Part model, mm, in its own coordinate system. Face numbers are marked on the shaded views. A direction names the side the tool comes from. Give positions to 0.01 mm unless a question says otherwise; leave off trailing zeros. Order: outer loops, then holes, each group sorted by start corner. A loop starts at its lowest first (then second) coordinate and runs counter-clockwise, first axis right, second up.
1. Mould opens along X. For the marked faces 3, 4, 5 and 6 say: +X half, -X half, draft (parallel to the pull), parting line (faces both ways), or undercut.
2. Slice it at C-C on x = 0. List the corners of the cut face in (y, z), and give its area (3 significant figures).
3. Probe line 1 (Z direction, x = 39, y = 9.25); line 2 (Z direction, x = -37.5, y = 12.5); line 3 (X direction, y = 13.25, z = -40). List the from-to ranges inside material, lowest first.
4. Slice it at B-B on z = 0. List the corners of the cut face in (x, y).
5. Drop flat-ended pins along their axis: pin 1 Ø5 at (y, z) = (11, 12) entering from +X; pin 2 Ø0.8 at (x, y) = (2, 0.5) entering from +Z; pin 3 Ø3 at (y, z) = (10, 5) entering from +X; pin 4 Ø0.8 at (y, z) = (1, 2.5) entering from +X. Give the stop position or say it passes through.
6. Which spindle directions (+Z, -Z, +X, -X, +Y, -Y) get a long thin tool onto all of the face, cutting with end or side? Do the marked faces 1 and 2. Say none if no direction does.
7. Slice it at A-A on y = 10.75. Give the number of separate pieces and of enclosed holes in the cut face, and give its area (3 significant figures).
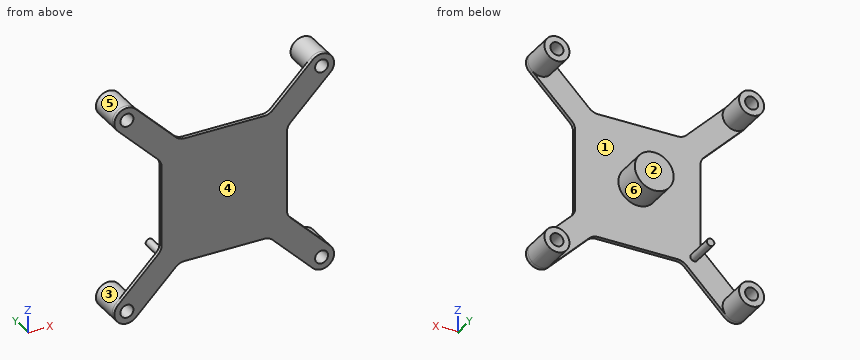
from build123d import *

# Parameters (mm, degrees)
SKETCH1_W           = 50
SKETCH1_H           = 50
SKETCH1_R           = 8
BOSS_EXTRUDE1_DEPTH = 1.5
BOSS_EXTRUDE3_START = -1.5
SKETCH5_R           = 2.6
SKETCH5_R_2         = 8
BOSS_EXTRUDE3_DEPTH = 1.5
FILLET1_R           = 5
SKETCH6_R           = 5
SKETCH6_R_2         = 2.6
BOSS_EXTRUDE4_DEPTH = 12
SKETCH7_R           = 8.25
BOSS_EXTRUDE5_DEPTH = 1.5
SKETCH8_R           = 7.75
BOSS_EXTRUDE6_DEPTH = 12
SKETCH9_R           = 1.5
BOSS_EXTRUDE7_DEPTH = 12


with BuildPart() as part:
    # Sketch1 → Boss-Extrude1 (new body)
    with BuildSketch(Plane(origin=(0, 0, 0), x_dir=(1, 0, 0), z_dir=(0, 1, 0))):
        Rectangle(SKETCH1_W, SKETCH1_H)
        with Locations(Location((0, 0, 0), (0, 0, 270))):
            Circle(SKETCH1_R, mode=Mode.SUBTRACT)
    extrude(amount=BOSS_EXTRUDE1_DEPTH)

    # Sketch5 → Boss-Extrude3 (add)
    with BuildSketch(Plane(origin=(0, 1.5, 0), x_dir=(1, 0, 0), z_dir=(0, 1, 0)).offset(BOSS_EXTRUDE3_START)):
        Polygon((-42.426406871, -35.355339059), (-25, -17.928932188), (-25, 17.928932188), (-42.426406871, 35.355339059), (-45.961940777, 38.890872965), (-38.890872965, 45.961940777), (-35.355339059, 42.426406871), (-17.928932188, 25), (17.928932188, 25), (35.355339059, 42.426406871), (38.890872965, 45.961940777), (45.961940777, 38.890872965), (42.426406871, 35.355339059), (25, 17.928932188), (25, -17.928932188), (42.426406871, -35.355339059), (45.961940777, -38.890872965), (38.890872965, -45.961940777), (35.355339059, -42.426406871), (17.928932188, -25), (-17.928932188, -25), (-35.355339059, -42.426406871), (-38.890872965, -45.961940777), (-45.961940777, -38.890872965), align=None)
        with Locations(Location((-38.890872965, -38.890872965, 0), (0, 0, 270))):
            Circle(SKETCH5_R, mode=Mode.SUBTRACT)
        with Locations(Location((38.890872965, 38.890872965, 0), (0, 0, 270))):
            Circle(SKETCH5_R, mode=Mode.SUBTRACT)
        with Locations(Location((38.890872965, -38.890872965, 0), (0, 0, 90))):
            Circle(SKETCH5_R, mode=Mode.SUBTRACT)
        with Locations(Location((-38.890872965, 38.890872965, 0), (0, 0, 90))):
            Circle(SKETCH5_R, mode=Mode.SUBTRACT)
        with Locations(Location((0, 0, 0), (0, 0, 270))):
            Circle(SKETCH5_R_2, mode=Mode.SUBTRACT)
    extrude(amount=BOSS_EXTRUDE3_DEPTH)

    # Fillet1
    fillet1_edges = [part.edges().sort_by_distance(p)[0] for p in [
        (17.928932188, 0.75, 25),
        (38.890872965, 0.75, 45.961940777),
        (45.961940777, 0.75, 38.890872965),
        (25, 0.75, 17.928932188),
        (25, 0.75, -17.928932188),
        (45.961940777, 0.75, -38.890872965),
        (38.890872965, 0.75, -45.961940777),
        (17.928932188, 0.75, -25),
        (-17.928932188, 0.75, -25),
        (-38.890872965, 0.75, -45.961940777),
        (-45.961940777, 0.75, -38.890872965),
        (-25, 0.75, -17.928932188),
        (-25, 0.75, 17.928932188),
        (-45.961940777, 0.75, 38.890872965),
        (-38.890872965, 0.75, 45.961940777),
        (-17.928932188, 0.75, 25),
    ]]
    fillet(fillet1_edges, radius=FILLET1_R - 0.0001)  # a hair under: the kernel refuses the full size

    # Sketch6 → Boss-Extrude4 (add)
    # profile 1 of 4: a face of its own
    with BuildSketch(Plane(origin=(0, 1.5, 0), x_dir=(1, 0, 0), z_dir=(0, 1, 0))):
        with Locations(Location((-38.890872965, -38.890872965, 0), (0, 0, 270))):
            Circle(SKETCH6_R)
        with Locations(Location((-38.890872965, -38.890872965, 0), (0, 0, 270))):
            Circle(SKETCH6_R_2, mode=Mode.SUBTRACT)
    # profile 2 of 4: a face of its own
    with BuildSketch(Plane(origin=(0, 1.5, 0), x_dir=(1, 0, 0), z_dir=(0, 1, 0))):
        with Locations(Location((-38.890872965, 38.890872965, 0), (0, 0, 270))):
            Circle(SKETCH6_R)
        with Locations(Location((-38.890872965, 38.890872965, 0), (0, 0, 270))):
            Circle(SKETCH6_R_2, mode=Mode.SUBTRACT)
    # profile 3 of 4: a face of its own
    with BuildSketch(Plane(origin=(0, 1.5, 0), x_dir=(1, 0, 0), z_dir=(0, 1, 0))):
        with Locations(Location((38.890872965, 38.890872965, 0), (0, 0, 270))):
            Circle(SKETCH6_R)
        with Locations(Location((38.890872965, 38.890872965, 0), (0, 0, 270))):
            Circle(SKETCH6_R_2, mode=Mode.SUBTRACT)
    # profile 4 of 4: a face of its own
    with BuildSketch(Plane(origin=(0, 1.5, 0), x_dir=(1, 0, 0), z_dir=(0, 1, 0))):
        with Locations(Location((38.890872965, -38.890872965, 0), (0, 0, 270))):
            Circle(SKETCH6_R)
        with Locations(Location((38.890872965, -38.890872965, 0), (0, 0, 270))):
            Circle(SKETCH6_R_2, mode=Mode.SUBTRACT)
    extrude(amount=BOSS_EXTRUDE4_DEPTH)

    # Sketch7 → Boss-Extrude5 (add)
    with BuildSketch(Plane(origin=(0, 1.5, 0), x_dir=(1, 0, 0), z_dir=(0, 1, 0))):
        Circle(SKETCH7_R)
    extrude(amount=-BOSS_EXTRUDE5_DEPTH)

    # Sketch8 → Boss-Extrude6 (add)
    with BuildSketch(Plane(origin=(0, 1.5, 0), x_dir=(1, 0, 0), z_dir=(0, 1, 0))):
        with Locations(Location((0, 0, 0), (0, 0, 90))):
            Circle(SKETCH8_R)
    extrude(amount=BOSS_EXTRUDE6_DEPTH)

    # Sketch9 → Boss-Extrude7 (add)
    with BuildSketch(Plane(origin=(0, 1.5, 0), x_dir=(1, 0, 0), z_dir=(0, 1, 0))):
        with Locations(Location((-22.5, 22.5, 0), (0, 0, 90))):
            Circle(SKETCH9_R)
    extrude(amount=BOSS_EXTRUDE7_DEPTH)


solid = part.part
Data:
1. face 3: undercut
1. face 4: draft
1. face 5: undercut
1. face 6: parting line
2. outline: (0, -25) - (1.5, -25) - (1.5, -7.75) - (13.5, -7.75) - (13.5, 7.75) - (1.5, 7.75) - (1.5, 25) - (0, 25) - close
2. area: 261 mm2
3. line 1: z = -43.89 to -41.49, -36.29 to -33.89, 33.89 to 36.29, 41.49 to 43.89
3. line 2: z = -43.69 to -41.09, -36.69 to -34.09, 34.09 to 36.69, 41.09 to 43.69
3. line 3: x = -43.77 to -41.24, -36.54 to -34.02, 34.02 to 36.54, 41.24 to 43.77
4. outline: (-25, 0) - (25, 0) - (25, 1.5) - (7.75, 1.5) - (7.75, 13.5) - (-7.75, 13.5) - (-7.75, 1.5) - (-25, 1.5) - close
5. pin 1: passes through
5. pin 2: stops at z = 25
5. pin 3: stops at x = 6.91
5. pin 4: stops at x = 25
6. face 1: +Y
6. face 2: +Z, -Z, +X, -X, +Y
7. separate pieces: 6
7. enclosed holes: 4
7. area: 425 mm2
